```python
from build123d import *

# Parameters (mm, degrees)
ESBO_O1_R                   = 1.65
RESSALTO_EXTRUS_O1_DEPTH    = 17
CORTE_EXTRUS_O2_DEPTH       = 32.941352507
CORTE_EXTRUS_O3_DEPTH       = 5.5
CORTE_EXTRUS_O4_DEPTH       = 15.3
CORTE_EXTRUS_O5_DEPTH       = 4.3
ESBO_O6_R                   = 12.5
ESBO_O7_R                   = 6.25
ESBO_O8_R                   = 6.25
RESSALTO_EXTRUS_O2_DEPTH    = 0.3
CORTE_EXTRUS_O6_DEPTH       = 32.941352507
CORTE_EXTRUS_O7_DEPTH       = 43.175111144
CORTE_EXTRUS_O7_DEPTH_BACK  = 43.175111144
ESBO_O10_R                  = 2.25
CORTE_EXTRUS_O14_DEPTH      = 34.222582739
CORTE_EXTRUS_O14_DEPTH_BACK = 34.222582739
CORTE_EXTRUS_O17_DEPTH      = 42.686958439
CORTE_EXTRUS_O17_DEPTH_BACK = 42.686958439
CORTE_EXTRUS_O18_DEPTH      = 1.5
ESBO_O22_W                  = 73.531346764
ESBO_O22_H                  = 29.602386944
CORTE_EXTRUS_O19_DEPTH      = 2
ESBO_O28_W                  = 27
ESBO_O28_H                  = 13.3
CORTE_EXTRUS_O22_DEPTH      = 10.5
ESBO_O27_R                  = 1.75
CORTE_EXTRUS_O23_DEPTH      = 42.686958439
CORTE_EXTRUS_O24_DEPTH      = 3


with BuildPart() as part:
    # Esboço1 → Ressalto-extrusão1 (new body)
    with BuildSketch(Plane(origin=(0, 0, 0), x_dir=(1, 0, 0), z_dir=(0, 1, 0))):
        with BuildLine():
            Line((-18.5, -15), (18.5, -15))
            ThreePointArc((18.5, -15), (21.328427125, -13.828427125), (22.5, -11))
            Line((22.5, -11), (22.5, 11))
            ThreePointArc((22.5, 11), (21.328427125, 13.828427125), (18.5, 15))
            Line((18.5, 15), (-18.5, 15))
            ThreePointArc((-18.5, 15), (-21.328427125, 13.828427125), (-22.5, 11))
            Line((-22.5, 11), (-22.5, -11))
            ThreePointArc((-22.5, -11), (-21.328427125, -13.828427125), (-18.5, -15))
        make_face()
        with Locations(Location((-17.5, -11, 0), (0, 0, 270))):
            Circle(ESBO_O1_R, mode=Mode.SUBTRACT)
        with Locations(Location((-17.5, 11, 0), (0, 0, 270))):
            Circle(ESBO_O1_R, mode=Mode.SUBTRACT)
        with Locations(Location((17.5, -11, 0), (0, 0, 270))):
            Circle(ESBO_O1_R, mode=Mode.SUBTRACT)
        with Locations(Location((17.5, 11, 0), (0, 0, 270))):
            Circle(ESBO_O1_R, mode=Mode.SUBTRACT)
    extrude(amount=RESSALTO_EXTRUS_O1_DEPTH)

    # Esboço3 → Corte-extrusão2 (cut, through all)
    with BuildSketch(Plane.XZ):
        with BuildLine():
            Line((-4, -15), (4, -15))
            Line((4, -15), (4, 0))
            ThreePointArc((4, 0), (0, 4), (-4, 0))
            Line((-4, 0), (-4, -15))
        make_face()
    extrude(amount=-CORTE_EXTRUS_O2_DEPTH, mode=Mode.SUBTRACT)

    # Esboço4 → Corte-extrusão3 (cut)
    with BuildSketch(Plane.XZ):
        with BuildLine():
            Line((-8.48, -15), (-8.48, 0))
            ThreePointArc((-8.48, 0), (0, 8.48), (8.48, 0))
            Line((8.48, 0), (8.48, -15))
            Line((8.48, -15), (-8.48, -15))
        make_face()
    extrude(amount=-CORTE_EXTRUS_O3_DEPTH, mode=Mode.SUBTRACT)

    # Esboço4<3> → Corte-extrusão4 (cut)
    with BuildSketch(Plane.XZ):
        with BuildLine():
            Line((-6.25, 0), (-6.25, -15))
            Line((-6.25, -15), (-4, -15))
            Line((-4, -15), (-4, 0))
            ThreePointArc((-4, 0), (0, 4), (4, 0))
            Line((4, 0), (4, -15))
            Line((4, -15), (6.25, -15))
            Line((6.25, -15), (6.25, 0))
            ThreePointArc((6.25, 0), (0, 6.25), (-6.25, 0))
        make_face()
    extrude(amount=-CORTE_EXTRUS_O4_DEPTH, mode=Mode.SUBTRACT)

    # Esboço5 → Corte-extrusão5 (cut)
    with BuildSketch(Plane.XZ.offset(-15.3)):
        with BuildLine():
            Line((-8.48, -15), (-8.48, 0.052643862))
            ThreePointArc((-8.48, 0.052643862), (0, 8.532643862), (8.48, 0.052643862))
            Line((8.48, 0.052643862), (8.48, -15))
            Line((8.48, -15), (-8.48, -15))
        make_face()
    extrude(amount=CORTE_EXTRUS_O5_DEPTH, mode=Mode.SUBTRACT)

    # Esboço6 → Loft1 section 0
    with BuildSketch(Plane(origin=(0, 17, 0), x_dir=(1, 0, 0), z_dir=(0, 1, 0))):
        Circle(ESBO_O6_R)
    # Esboço7 → Loft1 section 1
    with BuildSketch(Plane(origin=(0, 19, 0), x_dir=(1, 0, 0), z_dir=(0, 1, 0))):
        Circle(ESBO_O7_R)
    loft()

    # Esboço8 → Ressalto-extrusão2 (add)
    with BuildSketch(Plane(origin=(0, 19, 0), x_dir=(1, 0, 0), z_dir=(0, 1, 0))):
        with Locations(Location((0, 0, 0), (0, 0, 270))):
            Circle(ESBO_O8_R)
    extrude(amount=RESSALTO_EXTRUS_O2_DEPTH)

    # Esboço9 → Corte-extrusão6 (cut, through all)
    with BuildSketch(Plane.XZ.offset(-17)):
        with BuildLine():
            Line((-4, 0), (-3.999987243, -11.842772672))
            ThreePointArc((-3.999987243, -11.842772672), (2.212e-06, -12.500043117), (3.999990323, -11.842764489))
            Line((3.999990323, -11.842764489), (4, 0))
            ThreePointArc((4, 0), (0, 4), (-4, 0))
        make_face()
    extrude(amount=-CORTE_EXTRUS_O6_DEPTH, mode=Mode.SUBTRACT)

    # Esboço10 → Corte-extrusão7 (cut, two sides: drawn at the far end of the back side and taken through both)
    with BuildSketch(Plane(origin=(0, 0, -15), x_dir=(-1, 0, 0), z_dir=(0, 0, -1)).offset(-CORTE_EXTRUS_O7_DEPTH_BACK)):
        with Locations((0, 19.3)):
            Circle(ESBO_O10_R)
    extrude(amount=CORTE_EXTRUS_O7_DEPTH + CORTE_EXTRUS_O7_DEPTH_BACK, mode=Mode.SUBTRACT)

    # Esboço17 → Corte-extrusão14 (cut, two sides: drawn at the far end of the back side and taken through both)
    with BuildSketch(Plane.XZ.offset(-CORTE_EXTRUS_O14_DEPTH_BACK)):
        with BuildLine():
            Line((-8.48, -15), (8.48, -15))
            Line((8.48, -15), (18.5, -15))
            ThreePointArc((18.5, -15), (21.328427125, -13.828427125), (22.5, -11))
            Line((22.5, -11), (22.5, 11))
            ThreePointArc((22.5, 11), (21.328427125, 13.828427125), (18.5, 15))
            Line((18.5, 15), (-18.5, 15))
            ThreePointArc((-18.5, 15), (-21.328427125, 13.828427125), (-22.5, 11))
            Line((-22.5, 11), (-22.5, -11))
            ThreePointArc((-22.5, -11), (-21.328427125, -13.828427125), (-18.5, -15))
            Line((-18.5, -15), (-8.48, -15))
        make_face()
        with BuildLine():
            Line((8.48, -14.75), (18.5, -14.75))
            ThreePointArc((18.5, -14.75), (21.151650429, -13.651650429), (22.25, -11))
            Line((22.25, -11), (22.25, 11))
            ThreePointArc((22.25, 11), (21.151650429, 13.651650429), (18.5, 14.75))
            Line((18.5, 14.75), (-18.5, 14.75))
            ThreePointArc((-18.5, 14.75), (-21.151650429, 13.651650429), (-22.25, 11))
            Line((-22.25, 11), (-22.25, -11))
            ThreePointArc((-22.25, -11), (-21.151650429, -13.651650429), (-18.5, -14.75))
            Line((-18.5, -14.75), (-8.48, -14.75))
            Line((-8.48, -14.75), (8.48, -14.75))
        make_face(mode=Mode.SUBTRACT)
    extrude(amount=CORTE_EXTRUS_O14_DEPTH + CORTE_EXTRUS_O14_DEPTH_BACK, mode=Mode.SUBTRACT)

    # Esboço20 → Corte-extrusão17 (cut, two sides: drawn at the far end of the back side and taken through both)
    with BuildSketch(Plane.XY.offset(14.75).offset(-CORTE_EXTRUS_O17_DEPTH_BACK)):
        Polygon((-20.75, 0), (-22.25, 2.598076211), (-22.25, 0), align=None)
        Polygon((20.75, 0), (22.25, 2.598076211), (22.25, 0), align=None)
    extrude(amount=CORTE_EXTRUS_O17_DEPTH + CORTE_EXTRUS_O17_DEPTH_BACK, mode=Mode.SUBTRACT)

    # Esboço21 → Corte-extrusão18 (cut, symmetric)
    with BuildSketch(Plane(origin=(0, 8.25, 0), x_dir=(1, 0, 0), z_dir=(0, 1, 0))):
        Polygon((-20.848631561, 11), (-26.366704658, 20.557582963), (-21.343757316, 23.457582963), (-15.825684219, 13.9), (-14.151368439, 11), (-15.825684219, 8.1), (-19.174315781, 8.1), align=None)
        Polygon((19.174315781, 8.1), (20.848631561, 11), (26.085179504, 20.069967093), (21.158487208, 23.136685723), (15.825684219, 13.9), (14.151368439, 11), (15.825684219, 8.1), align=None)
        Polygon((15.825684219, -8.1), (14.151368439, -11), (15.825684219, -13.9), (19.678983152, -20.574109528), (25.513300663, -19.079443885), (20.848631561, -11), (19.174315781, -8.1), align=None)
        Polygon((-19.174315781, -8.1), (-20.848631561, -11), (-25.445111293, -18.961336431), (-20.050312904, -21.217271525), (-15.825684219, -13.9), (-14.151368439, -11), (-15.825684219, -8.1), align=None)
    extrude(amount=CORTE_EXTRUS_O18_DEPTH, both=True, mode=Mode.SUBTRACT)

    # Esboço22 → Corte-extrusão19 (cut)
    with BuildSketch(Plane.XZ):
        Rectangle(ESBO_O22_W, ESBO_O22_H)
    extrude(amount=-CORTE_EXTRUS_O19_DEPTH, mode=Mode.SUBTRACT)

    # Esboço28 → Corte-extrusão22 (cut)
    with BuildSketch(Plane(origin=(0, 0, -14.75), x_dir=(-1, 0, 0), z_dir=(0, 0, -1))):
        with Locations((0, 8.65)):
            Rectangle(ESBO_O28_W, ESBO_O28_H)
    extrude(amount=-CORTE_EXTRUS_O22_DEPTH, mode=Mode.SUBTRACT)

    # Esboço27 → Corte-extrusão23 (cut, through all)
    with BuildSketch(Plane(origin=(0, 0, -14.75), x_dir=(-1, 0, 0), z_dir=(0, 0, -1))):
        with Locations((-10.5, 8.25)):
            Circle(ESBO_O27_R)
        with Locations((10.5, 8.25)):
            Circle(ESBO_O27_R)
    extrude(amount=-CORTE_EXTRUS_O23_DEPTH, mode=Mode.SUBTRACT)

    # Esboço29 → Corte-extrusão24 (cut)
    with BuildSketch(Plane.XY.offset(14.75)):
        Polygon((-7.6, 9.924315781), (-10.5, 11.598631561), (-13.4, 9.924315781), (-13.4, 6.575684219), (-10.5, 4.901368439), (-7.6, 6.575684219), align=None)
        Polygon((10.5, 11.598631561), (7.6, 9.924315781), (7.6, 6.575684219), (10.5, 4.901368439), (13.4, 6.575684219), (13.4, 9.924315781), align=None)
    extrude(amount=-CORTE_EXTRUS_O24_DEPTH, mode=Mode.SUBTRACT)


solid = part.part
```
Part model, mm, in its own coordinate system. A direction names the side the tool comes from. Give positions to 0.01 mm unless a question says otherwise; leave off trailing zeros. Loops run counter-clockwise (first coordinate to the right, second up) from the corner with the lowest first, then second, coordinate; pieces in that order, holes last. Notation, with made-up numbers: M -38,75 L -33,75 A17 ccw -33,89 Z; hole C 7,33.5 d5. An arc over 180 degrees is marked long. Return JSON: item names as keys, results as strings.
1) Saw through at C-C, the plane x = 0. List the corners of the cut face in (y, z), then the cut area to 3 significant figures.
Calculated:
{"outline": "M 2,8.48 L 5.5,8.48 L 5.5,6.25 L 11,6.25 L 11,8.53 L 15.3,8.53 L 15.3,4 L 17.05,4 L 17.05,12.34 L 17,12.5 L 17,14.75 L 2,14.75 Z", "area": "114 mm2"}
2) Flat gauge pins, fed straight in: pin 1 Ø4.5 at (x, z) = (17.5, -11) entering from +Y; pin 2 Ø2.5 at (y, z) = (9, 13.5) entering from +X; pin 3 Ø1 at (x, y) = (8.5, 11.5) entering from -Z. Where does each tip first touch, or does it go through?
Calculated:
{"pin 1": "stops at y = 17", "pin 2": "stops at x = 22.04", "pin 3": "stops at z = -4.25"}
3) Pull direction Z, two halves, no side cores. Call faces 1 (the face through (-9.07, 5.727, 13.271)), 2 (the face through (-16.11, 4.34, 11.89)), 3 (the face through (0.14, 8.21, 6.25)): released by +Z, released by -Z, zero draft, split by the parting line, or undercut.
Calculated:
{"face 1": "zero draft", "face 2": "undercut", "face 3": "released by -Z"}
4) Saw through at D-D, the plane y = 8.25. Count the separate pieces of the cut face and the enclosed holes in it, then the cut area to 3 significant figures.
Calculated:
{"separate pieces": "3", "enclosed holes": "0", "area": "610 mm2"}
5) Drill centre lines: line 1 (X direction, y = 12.5, z = -11); line 2 (Z direction, x = 17.5, y = 12); line 3 (Y direction, x = -10.5, z = 10.5). Where is each one in solid material? Low to high.
Calculated:
{"line 1": "x = -22.25 to -19.15, -15.85 to -13.5, 13.5 to 15.85, 19.15 to 22.25", "line 2": "z = -14.75 to -12.65, -9.35 to 9.35, 12.65 to 14.75", "line 3": "y = 2 to 6.5, 10 to 17"}
6) 3-axis set-ups, long thin cutter, end or side, ignore diameter. For faces 4 (the face through (0, 17, 13)), 5 (the face through (4, 16, -7)), 6 (the face through (8.48, 4, -2)), 7 (the face through (12, 7, 11.75)), 8 (the face through (0.7, 11, 6.4)): which of +Z, -Z, +X, -X, +Y, -Y reach the whole face in a straight line?
Calculated:
{"face 4": "+Y", "face 5": "-Z, +Y, -Y", "face 6": "-Z, -Y", "face 7": "+Z", "face 8": "-Z"}
7) Saw through at B-B, the plane y = 12.25. List the corners of the cut face in (x, z), then the cut area to 3 significant figures.
Calculated:
{"outline": "M -22.25,-11 A3.75 ccw -18.5,-14.75 L -13.5,-14.75 L -13.5,-4.25 L -8.48,-4.25 L -8.48,0.05 A8.48 cw 8.48,0.05 L 8.48,-4.25 L 13.5,-4.25 L 13.5,-14.75 L 18.5,-14.75 A3.75 ccw 22.25,-11 L 22.25,11 A3.75 ccw 18.5,14.75 L -18.5,14.75 A3.75 ccw -22.25,11 Z; hole C -17.5,-11 d3.3; hole C -17.5,11 d3.3; hole C 17.5,-11 d3.3; hole C 17.5,11 d3.3", "area": "797 mm2"}
8) Saw through at A-A, the plane x = -17.5. List the corners of the cut face in (y, z).
Calculated:
{"outline": "M 2,-14.75 L 6.75,-14.75 L 6.75,-12.65 L 2,-12.65 Z; M 2,-9.35 L 6.75,-9.35 L 6.75,-8.1 L 9.75,-8.1 L 9.75,-9.35 L 17,-9.35 L 17,9.35 L 9.75,9.35 L 9.75,8.1 L 6.75,8.1 L 6.75,9.35 L 2,9.35 Z; M 2,12.65 L 6.75,12.65 L 6.75,14.75 L 2,14.75 Z; M 9.75,-14.75 L 17,-14.75 L 17,-12.65 L 9.75,-12.65 Z; M 9.75,12.65 L 17,12.65 L 17,14.75 L 9.75,14.75 Z"}
